Geometry check sheet. Reference: drawing and pictorial views, mm from the part's lowest x, y, z. A direction names the side the tool comes from. Coordinates: 2 decimals unless noted, no trailing zeros. Write each loop counter-clockwise with the first axis right and the second up, starting at its lowest first coordinate (ties: lowest second). Pieces come first, ordered by that corner, then holes. Notation, with made-up numbers: (20, 7) -> (77, 7) arc R30 cw to (77, 34) -> close; hole circle Ø7 at (10.5, -39.75). An arc over 180 degrees is marked (long way). Answer in a Markdown table with one row per item.
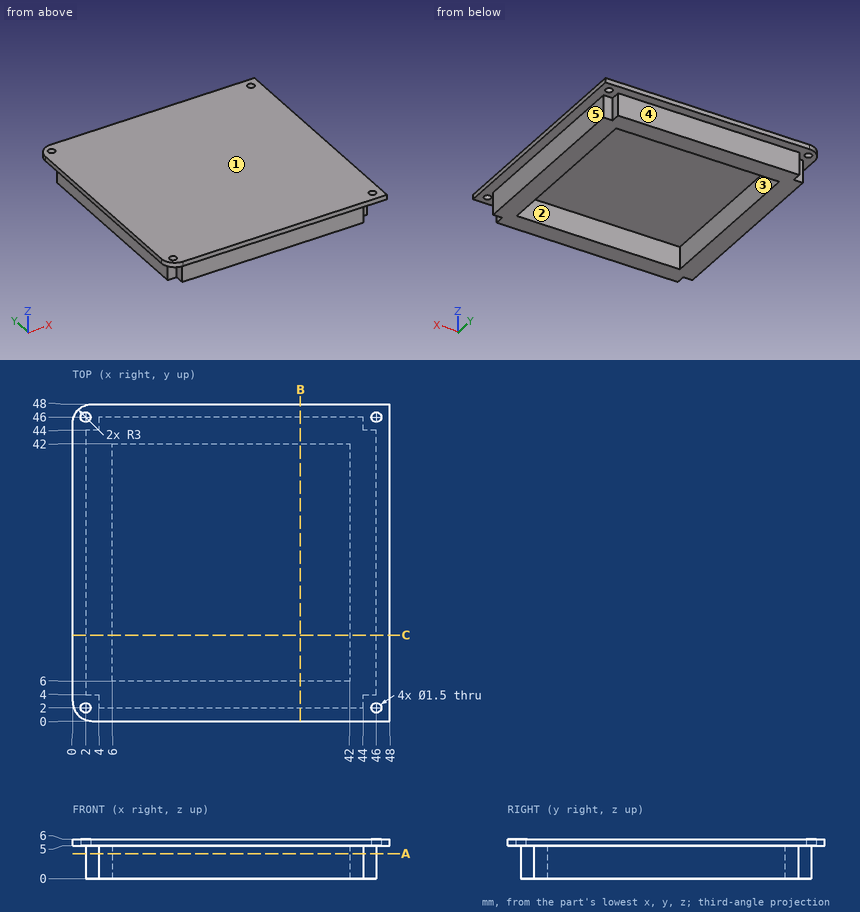
1. Mould release check, pull along Y, two halves, no side actions. Record for the marked faces 3, 4 and 5: released by +Y, released by -Y, zero draft, split by the parting line, or undercut.
Geometry says:
| item | result |
|---|---|
| face 3 | undercut |
| face 4 | released by +Y |
| face 5 | zero draft |
2. Tool access check on the marked faces 1 and 2. Record the directions out of +Z, -Z, +X, -X, +Y, -Y that give a thin tool (end or side, any length) a straight path to the whole face; none if there is none.
Geometry says:
| item | result |
|---|---|
| face 1 | +Z, +X, -X, +Y, -Y |
| face 2 | -Z |
3. Depth check by flat-ended pin: P1, Ø1.6, axis at x = 45.5, z = 2, coming from the +Y side; P2, Ø11, axis at x = 28, y = 30, coming from the -Z side; P3, Ø0.6, axis at y = 3, z = 1.5, coming from the +X side. Enter the tip coordinate at first touch or a pass-through.
Geometry says:
| item | result |
|---|---|
| P1 | y = 44 |
| P2 | z = 5 |
| P3 | x = 44 |
4. Section check A-A, the plane z = 3.8. Record the boundary of the cut face in (x, y).
Geometry says:
| item | result |
|---|---|
| outline | (2, 4) -> (4, 4) -> (4, 2) -> (44, 2) -> (44, 4) -> (46, 4) -> (46, 44) -> (44, 44) -> (44, 46) -> (4, 46) -> (4, 44) -> (2, 44) -> close; hole (6, 6) -> (42, 6) -> (42, 42) -> (6, 42) -> close |
5. Thickness scan on line 1 (X direction, y = 8, z = 2); line 2 (Y direction, x = 46, z = 5.7). Record the ranges inside material, lowest first. Write a range as from..to.
Geometry says:
| item | result |
|---|---|
| line 1 | 2..6, 42..46 |
| line 2 | 0..1.25, 2.75..45.25, 46.75..48 |
6. Section check B-B, the plane x = 34.5. Record the boundary of the cut face in (y, z), plus the area to 3 significant figures.
Geometry says:
| item | result |
|---|---|
| outline | (0, 5) -> (2, 5) -> (2, 0) -> (6, 0) -> (6, 5) -> (42, 5) -> (42, 0) -> (46, 0) -> (46, 5) -> (48, 5) -> (48, 6) -> (0, 6) -> close |
| area | 88.0 mm^2 |
